CAD build for the part. Positions are in the model's coordinates, mm. A direction names the side the tool comes from. Round coordinates to 2 decimals unless told otherwise and drop trailing zeros. Order: outer loops, then holes, each group sorted by start corner. A loop starts at its lowest first (then second) coordinate and runs counter-clockwise, first axis right, second up. Notation, with made-up numbers: (-3.75, 10) - (47.25, 10) arc R22 ccw to (47.25, 23) - close; hole circle Ø3 at (-15, 41.5). An arc over 180 degrees is marked (long way). Write item = value, one per line.
Autodesk Inventor part; units mm, degrees
ref_plane "YZ Plane" through (0, 0, 0) normal (1, 0, 0) x (0, 1, 0)
ref_plane "XZ Plane" through (0, 0, 0) normal (0, 1, 0) x (-1, 0, 0)
ref_plane "XY Plane" through (0, 0, 0) normal (0, 0, 1) x (1, 0, 0)
sketch "Esboço1" plane through (0, 0, 0) normal (1, 0, 0) x (0, 1, 0)
  line L0 (0, 0) -> (20, 0)
  line L1 (20, 0) -> (20, -132.9)
  line L2 (20, -132.9) -> (0, -132.9)
  line L3 (0, -132.9) -> (0, 0)
  line L4 (10, -132.9) -> (10, -62)
  circle A0 centre (10, -62) radius 2.5
  line L5 (10, -62) -> (10, -12)
  circle A1 centre (10, -12) radius 2.5
  dimension "d0" = 20
  dimension "d1" = 132.9
  dimension "d2" = 70.9
  dimension "d3" = 5
  dimension "d4" = 50
  dimension "d5" = 5
extrude "Extrusão1" add sketch "Esboço1" along normal blind 2
sketch "Esboço2" plane through (0, 0, 0) normal (0, 0, 1) x (1, 0, 0)
  line L0 (2, 20) -> (2, 0)
  line L1 (2, 0) -> (-2.5, 0)
  line L2 (-2.5, 0) -> (-2.5, 20)
  line L3 (-2.5, 20) -> (2, 20)
  line L4 (2, 20) -> (2, 0)
  point P0 (0, 0)
  dimension "d8" = 4.5
extrude "Extrusão2" add sketch "Esboço2" against normal blind 2
sketch "Esboço3" plane through (2, 0, 0) normal (1, 0, 0) x (0, 0, -1)
  circle A0 centre (62, 10) radius 2.5 construction
  line L0 (62, 10) -> (112, 10) construction
  point P0 (0, 0)
  dimension "d11" = 50
hole "Furo1" at (2, 10, -112) direction (-1, 0, 0) diameter 5 end through all
sketch "Esboço4" plane through (2, 0, 0) normal (1, 0, 0) x (0, 0, -1)
  circle A0 centre (12, 10) radius 2.5
  circle A1 centre (12, 10) radius 2.5
  point P0 (0, 0)
extrude "Extrusão3" add sketch "Esboço4" against normal blind 2
properties part number "Chapa da Caixa de Segurança"
(1) Band-saw the part on B-B on z = -62. List the corners of the cut face in (x, y), plus the area to 3 significant figures.
Solved:
outline = (0, 0) - (2, 0) - (2, 7.5) - (0, 7.5) - close; (0, 12.5) - (2, 12.5) - (2, 20) - (0, 20) - close
area = 30.0 mm²
(2) Band-saw the part on A-A on y = 10. List the corners of the cut face in (x, z), plus the area to 3 significant figures.
Solved:
outline = (-2.5, -2) - (0, -2) - (0, -59.5) - (2, -59.5) - (2, 0) - (-2.5, 0) - close; (0, -132.9) - (2, -132.9) - (2, -114.5) - (0, -114.5) - close; (0, -109.5) - (2, -109.5) - (2, -64.5) - (0, -64.5) - close
area = 251 mm²
(3) Probe line 1 along Z through (x, y) = (0.6, 10); line 2 along Y through (x, z) = (0.65, -62); line 3 along X through (y, z) = (12.5, -21). List the from-to ranges inside material, lowest first.
Solved:
line_1 = -132.9 to -114.5, -109.5 to -64.5, -59.5 to 0
line_2 = 0 to 7.5, 12.5 to 20
line_3 = 0 to 2
(4) Tool access for faces 1 (the flat face through (0, 10, -67)), 2 (the cylindrical face through (0.99, 9.67, -64.48)): list every direction of +Z, -Z, +X, -X, +Y, -Y with a clear straight run to the whole face (end or side of a thin tool).
Solved:
face_1 = -Z, -X, +Y, -Y
face_2 = +X, -X
(5) Band-saw the part on D-D on x = -1.35. List the corners of the cut face in (y, z), plus the area to 3 significant figures.
Solved:
outline = (0, -2) - (20, -2) - (20, 0) - (0, 0) - close
area = 40.0 mm²
(6) Band-saw the part on C-C on y = 16. List the corners of the cut face in (x, z), plus the area to 3 significant figures.
Solved:
outline = (-2.5, -2) - (0, -2) - (0, -132.9) - (2, -132.9) - (2, 0) - (-2.5, 0) - close
area = 271 mm²
(7) Drop flat-ended pins along their axis: pin 1 (1 mm diameter, centred on y = 6.5, z = -35.5, fed in from -X); pin 2 (1.2 mm diameter, centred on x = -1.5, y = 13.5, fed in from -Z). Give the stop position or say it passes through.
Solved:
pin_1 = 0
pin_2 = -2
